Design review of the part built by this model. Coordinates are the model's own, in mm. A direction names the side the tool comes from. Give positions to 0.01 mm unless a question says otherwise; leave off trailing zeros. Write each loop counter-clockwise with the first axis right and the second up, starting at its lowest first coordinate (ties: lowest second). Pieces come first, ordered by that corner, then holes. Notation, with made-up numbers: (29, 26) -> (51, 26) arc R26 cw to (51, 42) -> close; hole circle Ø1 at (-9, -30). An arc over 180 degrees is marked (long way). Use CSV: the item, a comma, the result in double quotes.
```python
from build123d import *

# Parameters (mm, degrees)
SKETCH_1_W                   = 60
SKETCH_1_H                   = 130
EXTRUDE_1_DEPTH              = 5
HOLE_WIZARD_M3_1_D           = 3.4
HOLE_WIZARD_M3_1_DEPTH       = 7.5
HOLE_WIZARD_M3_1_CSINK_D     = 6.3
HOLE_WIZARD_M3_1_CSINK_ANGLE = 90
HOLE_WIZARD_M3_1_TIP         = 1.021463052
SKETCH_6_R                   = 12.5
CUT_EXTRUDE_1_DEPTH          = 72.763500472
F_1_0MM_2_AT_2_COUNT         = 2
F_1_0MM_2_AT_2_PITCH         = 25
F_1_0MM_2_AT_3_COUNT         = 2
F_1_0MM_2_AT_3_PITCH         = 50
F_1_0MM_1_D                  = 2.2
SKETCH_13_R                  = 6
CUT_EXTRUDE_2_DEPTH          = 72.763500472


with BuildPart() as part:
    # 草圖1 → 填料-伸長1 (new body)
    with BuildSketch(Plane(origin=(0, 0, 0), x_dir=(1, 0, 0), z_dir=(0, 1, 0))):
        Rectangle(SKETCH_1_W, SKETCH_1_H)
    extrude(amount=EXTRUDE_1_DEPTH)

    # M3 錐坑平頭螺釘的錐孔1
    with Locations(Plane(origin=(0, 5, 0), x_dir=(1, 0, 0), z_dir=(0, 1, 0))):
        with Locations((-15.5, 12.5), (-15.5, -18.5), (15.5, 12.5), (15.5, -18.5)):
            CounterSinkHole(HOLE_WIZARD_M3_1_D / 2, HOLE_WIZARD_M3_1_CSINK_D / 2, depth=HOLE_WIZARD_M3_1_DEPTH, counter_sink_angle=HOLE_WIZARD_M3_1_CSINK_ANGLE)
            with Locations((0, 0, -(HOLE_WIZARD_M3_1_DEPTH + HOLE_WIZARD_M3_1_TIP / 2))):  # 118° drill point
                Cone(0, HOLE_WIZARD_M3_1_D / 2, HOLE_WIZARD_M3_1_TIP, mode=Mode.SUBTRACT)

    # 草圖6 → 除料-伸長1 (cut, through all)
    with BuildSketch(Plane(origin=(0, 5, 0), x_dir=(1, 0, 0), z_dir=(0, 1, 0))):
        with Locations(Location((0, -3, 0), (0, 0, 270))):
            Circle(SKETCH_6_R)
    extrude(amount=-CUT_EXTRUDE_1_DEPTH, mode=Mode.SUBTRACT)

    # 草圖8 → Ø1.0mm 定位孔2 (revolve, cut)
    with BuildSketch(Plane(origin=(25, 2.5, -65), x_dir=(0, 1, 0), z_dir=(1, 0, 0))):
        Polygon((0, 0), (0, 8.311161836), (1.35, 7.5), (1.35, 0), align=None)
    f_1_0mm_2 = revolve(axis=Axis((25, 2.5, -71.35), (0, 0, 1)), mode=Mode.SUBTRACT)

    # Ø1.0mm 定位孔2 at 2: Ø1.0mm 定位孔2 ×2
    with Locations(*[(-i * F_1_0MM_2_AT_2_PITCH, 0, 0) for i in range(1, F_1_0MM_2_AT_2_COUNT)]):
        add(f_1_0mm_2, mode=Mode.SUBTRACT)

    # Ø1.0mm 定位孔2 at 3: Ø1.0mm 定位孔2 ×2
    with Locations(*[(-i * F_1_0MM_2_AT_3_PITCH, 0, 0) for i in range(1, F_1_0MM_2_AT_3_COUNT)]):
        add(f_1_0mm_2, mode=Mode.SUBTRACT)

    # 鏡射1: Ø1.0mm 定位孔2 across plane
    add(f_1_0mm_2.mirror(Plane.XY), mode=Mode.SUBTRACT)

    # 鏡射1 copy 1 sketch → 鏡射1 copy 1 (revolve, cut)
    with BuildSketch(Plane(origin=(0, 2.5, 65), x_dir=(0, 1, 0), z_dir=(1, 0, 0))):
        Polygon((0, 0), (0, -8.311161836), (1.35, -7.5), (1.35, 0), align=None)
    revolve(axis=Axis((0, 2.5, 71.35), (0, 0, 1)), mode=Mode.SUBTRACT)

    # 鏡射1 copy 2 sketch → 鏡射1 copy 2 (revolve, cut)
    with BuildSketch(Plane(origin=(-25, 2.5, 65), x_dir=(0, 1, 0), z_dir=(1, 0, 0))):
        Polygon((0, 0), (0, -8.311161836), (1.35, -7.5), (1.35, 0), align=None)
    revolve(axis=Axis((-25, 2.5, 71.35), (0, 0, 1)), mode=Mode.SUBTRACT)

    # Ø1.0mm 定位孔1 (through all)
    with Locations(Plane(origin=(0, 5, 0), x_dir=(1, 0, 0), z_dir=(0, 1, 0))):
        with Locations((0, 32.5), (0, 14)):
            Hole(F_1_0MM_1_D / 2)

    # 草圖13 → 除料-伸長2 (cut, through all)
    with BuildSketch(Plane(origin=(0, 5, 0), x_dir=(1, 0, 0), z_dir=(0, 1, 0))):
        with Locations(Location((0, 23, 0), (0, 0, 270))):
            Circle(SKETCH_13_R)
    extrude(amount=-CUT_EXTRUDE_2_DEPTH, mode=Mode.SUBTRACT)


solid = part.part
```
(1) For line 1 along X through (y, z) = (2.45, 18.5); line 2 along Z through (x, y) = (-15.5, 2.25); line 3 along X through (y, z) = (2.5, 63), list the stretches that pass through material, from the lowest coordinate up. Write a range as [from, to].
Established:
line 1,"x = [-30, -17.2], [-13.8, 13.8], [17.2, 30]"
line 2,"z = [-65, -14.2], [-10.8, 16.8], [20.2, 65]"
line 3,"x = [-30, -26.35], [-23.65, -1.35], [1.35, 23.65], [26.35, 30]"
(2) Tool access review of faces 4 (the face through (0.82, 1.43, 61.3)), 5 (the face through (1.2, 3.12, -61.3)), 6 (the face through (-0.59, 2.47, -33.43)): name each direction out of +Z, -Z, +X, -X, +Y, -Y from which nothing blocks a thin tool from reaching the whole face with its end or side.
Established:
face 4,"+Z"
face 5,"-Z"
face 6,"+Y, -Y"
(3) Take a section at C-C (x = -7.5). Write out the cut boundary in (y, z), then the cut area to 3 significant figures.
Established:
outline,"(0, -65) -> (5, -65) -> (5, -7) -> (0, -7) -> close; (0, 13) -> (5, 13) -> (5, 65) -> (0, 65) -> close"
area,"550 mm2"
(4) Clearance check with flat-ended pins moving along their axes: pin 1 (2 mm diameter, centred on x = 25, y = 2.5, fed in from +Z); pin 2 (2.5 mm diameter, centred on x = -25, y = 2.5, fed in from +Z); pin 3 (1.6 mm diameter, centred on x = 0, y = 2.5, fed in from +Z). State where each tip first meets the part, or that it passes through.
Established:
pin 1,"stops at z = 57.29"
pin 2,"stops at z = 57.44"
pin 3,"stops at z = 57.17"
(5) Take a section at D-D (x = 15.5). Write out the cut boundary in (y, z).
Established:
outline,"(0, -65) -> (5, -65) -> (5, -15.65) -> (3.55, -14.2) -> (0, -14.2) -> close; (0, -10.8) -> (3.55, -10.8) -> (5, -9.35) -> (5, 15.35) -> (3.55, 16.8) -> (0, 16.8) -> close; (0, 20.2) -> (3.55, 20.2) -> (5, 21.65) -> (5, 65) -> (0, 65) -> close"
(6) Take a section at A-A (z = 3). Write out the cut boundary in (x, y).
Established:
outline,"(-30, 0) -> (-12.5, 0) -> (-12.5, 5) -> (-30, 5) -> close; (12.5, 0) -> (30, 0) -> (30, 5) -> (12.5, 5) -> close"
(7) Mouldability with a two-part tool opening along X and no side actions: class faces 1 (the face through (13.88, 1.75, 17.99)), 2 (the face through (-0.4, 0.8, 65)), 3 (the face through (-30, 2, 1)) as +X half, -X half, draft (parallel to the pull), parting line (faces both ways), or undercut.
Established:
face 1,"undercut"
face 2,"draft"
face 3,"-X half"
(8) Take a section at B-B (z = 18.5). Write out the cut boundary in (x, y).
Established:
outline,"(-30, 0) -> (-17.2, 0) -> (-17.2, 3.55) -> (-18.65, 5) -> (-30, 5) -> close; (-13.8, 0) -> (13.8, 0) -> (13.8, 3.55) -> (12.35, 5) -> (-12.35, 5) -> (-13.8, 3.55) -> close; (17.2, 0) -> (30, 0) -> (30, 5) -> (18.65, 5) -> (17.2, 3.55) -> close"
